Design review of the part built by this model. Coordinates are the model's own, in mm. Round coordinates to 2 decimals unless told otherwise and drop trailing zeros. Write each loop counter-clockwise with the first axis right and the second up, starting at its lowest first coordinate (ties: lowest second). Pieces come first, ordered by that corner, then holes. Notation, with made-up numbers: (22.25, 53.5) -> (31.25, 53.5) arc R18 ccw to (31.25, 84.5) -> close; hole circle Ø1 at (40.25, 82.5). An arc over 180 degrees is marked (long way). Write item = value, one per line. Start each with the question number.
Item 1: Add section A-A, the plane y = -1.05. State the section outline as (x, z) points.
Item 2: Add section B-B, the plane y = -0.4. State the section outline as (x, z) points, then the cut area to 3 significant figures.
Item 3: For pin 1 Ø1 at (y, z) = (-1, -3.5) entering from +X; pin 2 Ø1 at (y, z) = (0, -2.5) entering from -X; pin 3 Ø1 at (y, z) = (-1, 3.5) entering from -X, all flat-tipped, find the tip position at first contact; note any pin that passes through.
Item 4: To check wall thickness, follow L1, parallel to X at y = 1.85, z = 0; L2, parallel to X at y = -1.3, z = 0; L3, parallel to Y at x = 0.5, z = 3. State the ranges of each line that lie inside material, in increasing order.
from build123d import *

# Parameters (mm, degrees)
CHAMFER1_SIZE = 0.1


with BuildPart() as part:
    # Sketch1 → Revolve1 (revolve)
    with BuildSketch(Plane(origin=(0, 0, 0), x_dir=(0, 0, -1), z_dir=(1, 0, 0))):
        Polygon((4.6, 0), (6, 1.4), (6, 2), (1.5, 2), (1.5, -2), (6, -2), (6, -1.4), align=None)
    revolve(axis=Axis((0, 2, 0), (0, -1, 0)))

    # Sketch3 → Cut-Revolve2 (revolve, cut)
    with BuildSketch(Plane(origin=(0, 0, 0), x_dir=(0, 0, -1), z_dir=(1, 0, 0))):
        Polygon((3.3, 1.8), (3.5, 1.7), (3.5, 2), (2.25, 2), (2.25, 1.7), (2.45, 1.8), align=None)
    cut_revolve2 = revolve(axis=Axis((0, 2, 0), (0, -1, 0)), mode=Mode.SUBTRACT)

    # Mirror1: Cut-Revolve2 across plane
    add(cut_revolve2.mirror(Plane.ZX), mode=Mode.SUBTRACT)

    # Chamfer1
    chamfer1_edges = [part.edges().sort_by_distance(p)[0] for p in [
        (0, 2, 3.5),
        (0, 2, 2.25),
        (0, -2, 3.5),
        (0, -2, 2.25),
        (0, 2, 6),
        (0, -2, 6),
        (0, -2, 1.5),
        (0, 2, 1.5),
    ]]
    chamfer(chamfer1_edges, length=CHAMFER1_SIZE)


solid = part.part
Result set:
q1.outline = circle Ø11.3 at (0, 0); hole circle Ø3 at (0, 0)
q2.outline = circle Ø10 at (0, 0); hole circle Ø3 at (0, 0)
q2.area = 71.5 mm²
q3.pin_1 = 5.08
q3.pin_2 = -4.51
q3.pin_3 = -5.08
q4.L1 = -6 to -3.5, -2.25 to -1.5, 1.5 to 2.25, 3.5 to 6
q4.L2 = -5.9 to -1.5, 1.5 to 5.9
q4.L3 = -1.8 to 1.8
